The figure shows three views and two pictorial views of one solid part (mm, origin at its lowest corner). Answer the questions. Round coordinates to 2 decimals unless told otherwise and drop trailing zeros. Loops run counter-clockwise (first coordinate to the right, second up) from the corner with the lowest first, then second, coordinate; pieces in that order, holes last. Notation, with made-up numbers: (-3, 45) -> (21, 45) arc R25 ccw to (21, 63) -> close; hole circle Ø3 at (61.5, -1). An arc over 180 degrees is marked (long way). Write item = value, one per line. Start each with the question number.
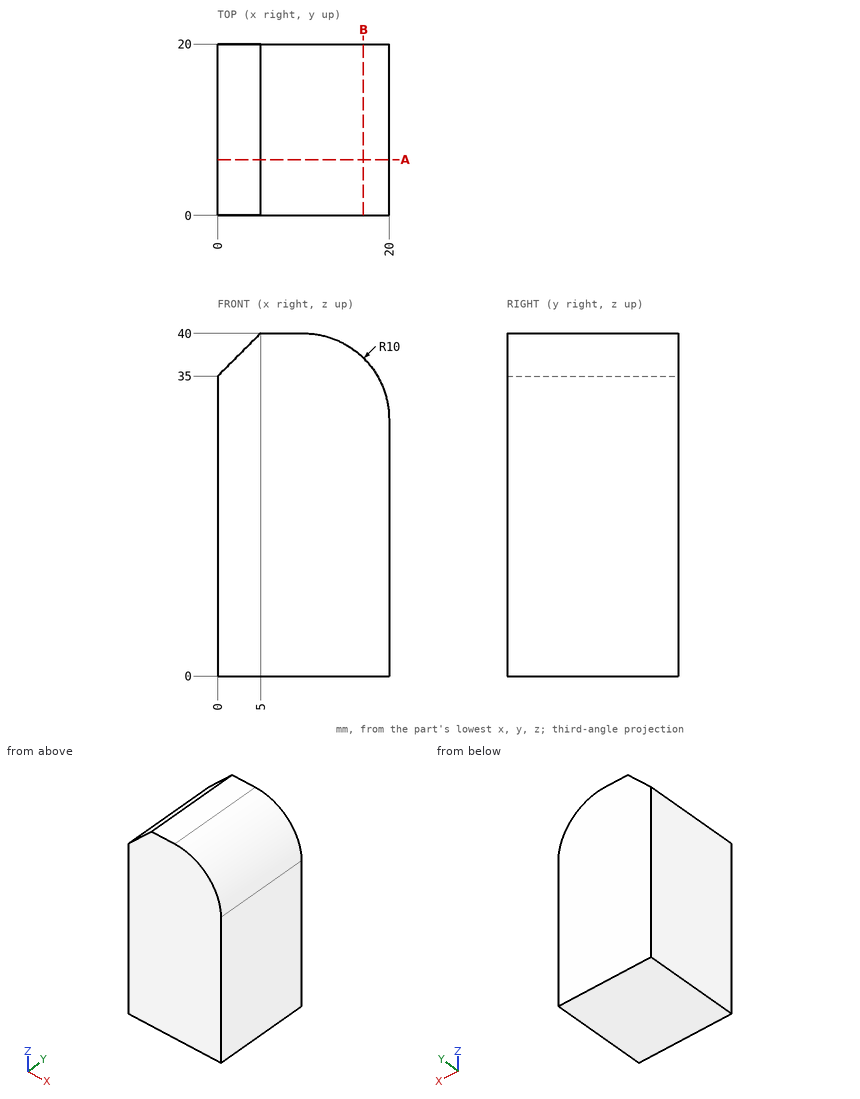
Item 1: Section A-A (y = 6.5) is taken. Determine the outline of the cut face in (x, z), then the cut area to 3 significant figures.
Item 2: Section B-B (x = 17) is taken. Determine the outline of the cut face in (y, z).
Item 3: Find the intervals of material crossed by line 1 along Z through (x, y) = (11.5, 1.75); line 2 along Z through (x, y) = (12.25, 15); line 3 along X through (y, z) = (10.5, 36.5), in increasing order. Write a range as [from, to].
Worked answers:
q1.outline = (0, 0) -> (20, 0) -> (20, 30) arc R10 ccw to (10, 40) -> (5, 40) -> (0, 35) -> close
q1.area = 766 mm2
q2.outline = (0, 0) -> (20, 0) -> (20, 37.14) -> (0, 37.14) -> close
q3.line_1 = [0, 39.89]
q3.line_2 = [0, 39.74]
q3.line_3 = [1.5, 17.6]
